```python
from build123d import *

# Parameters (mm, degrees)
Y_KSEKLIK_EKSTR_ZYON1_DEPTH = 56
RADYUS1_R                   = 10
IZIM2_R                     = 5
KES_EKSTR_ZYON1_DEPTH       = 130.760913174


with BuildPart() as part:
    # Çizim1 → Yükseklik-Ekstrüzyon1 (new body)
    with BuildSketch(Plane.XY):
        Polygon((-33.438372489, 12.291666667), (11.561627511, 12.291666667), (11.561627511, 24.291666667), (-27.438372489, 24.291666667), (-27.438372489, 26.291666667), (-77.438372489, 26.291666667), (-77.438372489, 24.291666667), (-116.438372489, 24.291666667), (-116.438372489, 12.291666667), (-71.438372489, 12.291666667), (-71.438372489, 16.291666667), (-33.438372489, 16.291666667), align=None)
    extrude(amount=Y_KSEKLIK_EKSTR_ZYON1_DEPTH)

    # Radyus1
    radyus1_edges = [part.edges().sort_by_distance(p)[0] for p in [
        (11.561627511, 18.291666667, 0),
        (-116.438372489, 18.291666667, 0),
        (11.561627511, 18.291666667, 56),
        (-116.438372489, 18.291666667, 56),
    ]]
    fillet(radyus1_edges, radius=RADYUS1_R)

    # Çizim2 → Kes-Ekstrüzyon1 (cut, through all)
    with BuildSketch(Plane(origin=(0, 24.291666667, 0), x_dir=(1, 0, 0), z_dir=(0, 1, 0))):
        with Locations(Location((-106.438372489, -11, 0), (0, 0, 180))):
            Circle(IZIM2_R)
        with Locations(Location((-106.438372489, -45, 0), (0, 0, 180))):
            Circle(IZIM2_R)
        with Locations(Location((1.561627511, -45, 0), (0, 0, 180))):
            Circle(IZIM2_R)
        with Locations(Location((1.561627511, -11, 0), (0, 0, 180))):
            Circle(IZIM2_R)
    extrude(amount=-KES_EKSTR_ZYON1_DEPTH, mode=Mode.SUBTRACT)


solid = part.part
```
Verification items for the finished model (mm, model axes). A direction names the side the tool comes from. Coordinates: 2 decimals unless noted, no trailing zeros. Loops run counter-clockwise (first coordinate to the right, second up) from the corner with the lowest first, then second, coordinate; pieces in that order, holes last. Notation, with made-up numbers: (84, -31.75) -> (142, -31.75) arc R19 ccw to (142, -17.75) -> close; hole circle Ø7 at (42.5, 52). An arc over 180 degrees is marked (long way). Answer in a Markdown table with one row per item.
1) Draft check along X on faces 1 (the face through (-71.438, 14, 28)), 2 (the face through (11.562, 18, 28)), 3 (the face through (-33.438, 14, 28)), 4 (the face through (-113.59, 18.21, 3.01)). Enter one of: released by +X, released by -X, zero draft, split by the parting line, or undercut.
The answers:
| item | result |
|---|---|
| face 1 | undercut |
| face 2 | released by +X |
| face 3 | undercut |
| face 4 | released by -X |
2) Depth check by flat-ended pin: P1, Ø13, axis at x = 1.56, z = 11, coming from the +Y side; P2, Ø19, axis at x = -47, z = 30.5, coming from the -Y side; P3, Ø0.6, axis at y = 25, z = 41, coming from the +X side; P4, Ø8, axis at x = -106.44, z = 11, coming from the +Y side (3 decimals). Enter the tip coordinate at first touch or a pass-through.
The answers:
| item | result |
|---|---|
| P1 | stops at y = 24.29 |
| P2 | stops at y = 16.29 |
| P3 | stops at x = -27.44 |
| P4 | passes through |
3) Section check B-B (y = 22.25). Record the cut outline in (x, z).
The answers:
| item | result |
|---|---|
| outline | (-116.44, 10) arc R10 ccw to (-106.44, 0) -> (1.56, 0) arc R10 ccw to (11.56, 10) -> (11.56, 46) arc R10 ccw to (1.56, 56) -> (-106.44, 56) arc R10 ccw to (-116.44, 46) -> close; hole circle Ø10 at (-106.44, 11); hole circle Ø10 at (-106.44, 45); hole circle Ø10 at (1.56, 11); hole circle Ø10 at (1.56, 45) |
4) Section check A-A (y = 14.5). Record the cut outline in (x, z).
The answers:
| item | result |
|---|---|
| outline | (-116.44, 10) arc R10 ccw to (-106.44, 0) -> (-71.44, 0) -> (-71.44, 56) -> (-106.44, 56) arc R10 ccw to (-116.44, 46) -> close; (-33.44, 0) -> (1.56, 0) arc R10 ccw to (11.56, 10) -> (11.56, 46) arc R10 ccw to (1.56, 56) -> (-33.44, 56) -> close; hole circle Ø10 at (-106.44, 11); hole circle Ø10 at (-106.44, 45); hole circle Ø10 at (1.56, 11); hole circle Ø10 at (1.56, 45) |
5) Access from +Z, -Z, +X, -X, +Y, -Y to the whole of each face (thin tool, end or side, straight path). Record for faces 5 (the face through (-97, 24.292, 28)), 6 (the face through (-8, 24.292, 28)), 7 (the face through (-53, 16.292, 28)).
The answers:
| item | result |
|---|---|
| face 5 | +Z, -Z, -X, +Y |
| face 6 | +Z, -Z, +X, +Y |
| face 7 | +Z, -Z, -Y |
6) Scan lines: line 1 along Z through (x, y) = (-106, 20.5); line 2 along Z through (x, y) = (-1, 17.75); line 3 along X through (y, z) = (14.75, 44). Record each from-to range of solid material in increasing order. Write a range as from..to.
The answers:
| item | result |
|---|---|
| line 1 | z = 0..6.02, 15.98..40.02, 49.98..56 |
| line 2 | z = 0..6.71, 15.29..40.71, 49.29..56 |
| line 3 | x = -116.44..-111.34, -101.54..-71.44, -33.44..-3.34, 6.46..11.56 |
7) Section check C-C (z = 8.5). Record the cut outline in (x, y), and give its area (3 significant figures).
The answers:
| item | result |
|---|---|
| outline | (-116.33, 12.29) -> (-110.77, 12.29) -> (-110.77, 24.29) -> (-116.33, 24.29) -> close; (-102.11, 12.29) -> (-71.44, 12.29) -> (-71.44, 16.29) -> (-33.44, 16.29) -> (-33.44, 12.29) -> (-2.77, 12.29) -> (-2.77, 24.29) -> (-27.44, 24.29) -> (-27.44, 26.29) -> (-77.44, 26.29) -> (-77.44, 24.29) -> (-102.11, 24.29) -> close; (5.89, 12.29) -> (11.45, 12.29) -> (11.45, 24.29) -> (5.89, 24.29) -> close |
| area | 1,270 mm2 |
8) Section check D-D (x = -105). Record the cut outline in (y, z), and give its area (3 significant figures).
The answers:
| item | result |
|---|---|
| outline | (12.29, 0) -> (24.29, 0) -> (24.29, 6.21) -> (12.29, 6.21) -> close; (12.29, 15.79) -> (24.29, 15.79) -> (24.29, 40.21) -> (12.29, 40.21) -> close; (12.29, 49.79) -> (24.29, 49.79) -> (24.29, 56) -> (12.29, 56) -> close |
| area | 442 mm2 |
